The listing builds one solid part. Answer for the finished solid, in the listing's coordinates (mm). Give positions to 0.01 mm unless a question says otherwise; leave off trailing zeros. Write each loop counter-clockwise with the first axis right and the second up, starting at its lowest first coordinate (ties: lowest second). Pieces come first, ordered by that corner, then holes.
```python
from build123d import *

# Parameters (mm, degrees)
SKETCH5_R           = 84.7725
SKETCH5_R_2         = 6.35
BOSS_EXTRUDE1_DEPTH = 6.35


with BuildPart() as part:
    # Sketch5 → Boss-Extrude1 (new body)
    with BuildSketch(Plane(origin=(0, 0, 0), x_dir=(1, 0, 0), z_dir=(0, 1, 0))):
        with BuildLine():
            Line((-108.51132569, 114.857435108), (257.591051155, 114.857435108))
            ThreePointArc((257.591051155, 114.857435108), (263.497362796, 112.410960723), (265.943837181, 106.504649083))
            Line((265.943837181, 106.504649083), (265.943837181, 22.684649083))
            ThreePointArc((265.943837181, 22.684649083), (263.497362796, 16.778337443), (257.591051155, 14.331863057))
            Line((257.591051155, 14.331863057), (240.397032386, 14.331863057))
            ThreePointArc((240.397032386, 14.331863057), (234.490720746, 11.885388672), (232.044246361, 5.979077032))
            Line((232.044246361, 5.979077032), (232.044246361, -98.583895379))
            ThreePointArc((232.044246361, -98.583895379), (229.597771976, -104.490207019), (223.691460335, -106.936681404))
            Line((223.691460335, -106.936681404), (-106.508539665, -106.936681404))
            ThreePointArc((-106.508539665, -106.936681404), (-112.414851305, -104.490207019), (-114.86132569, -98.583895379))
            Line((-114.86132569, -98.583895379), (-114.86132569, 108.507435108))
            ThreePointArc((-114.86132569, 108.507435108), (-113.001453751, 112.997563169), (-108.51132569, 114.857435108))
        make_face()
        Circle(SKETCH5_R, mode=Mode.SUBTRACT)
        with Locations((251.46, 89.968152547)):
            Circle(SKETCH5_R_2, mode=Mode.SUBTRACT)
        with Locations((251.46, 39.221145619)):
            Circle(SKETCH5_R_2, mode=Mode.SUBTRACT)
        with Locations((-95.238376165, -11.844376537)):
            Circle(SKETCH5_R_2, mode=Mode.SUBTRACT)
        with Locations((57.035275027, -75.64676797)):
            Circle(SKETCH5_R_2, mode=Mode.SUBTRACT)
        with Locations((36.152941234, 88.127278006)):
            Circle(SKETCH5_R_2, mode=Mode.SUBTRACT)
    extrude(amount=-BOSS_EXTRUDE1_DEPTH)


solid = part.part
```
Item 1: Consider probe 1 along Z at (x, y) = (251.46, -4.5); probe 2 along Z at (x, y) = (0, -3.5); probe 3 along Z at (x, y) = (35.5, -1.5). Determine where each line is inside the solid, lowest interval first.
Conclusion:
probe 1: z = -114.86 to -96.32, -83.62 to -45.57, -32.87 to -14.33
probe 2: z = -114.86 to -84.77, 84.77 to 106.94
probe 3: z = -114.86 to -94.44, -81.81 to -76.98, 76.98 to 106.94
Item 2: A cutting plane is placed at C-C, the plane z = 0. Give the vertices of the cut face in (x, y), plus the area to 3 significant figures.
Conclusion:
outline: (-114.86, -6.35) - (-84.77, -6.35) - (-84.77, 0) - (-114.86, 0) - close; (84.77, -6.35) - (232.04, -6.35) - (232.04, 0) - (84.77, 0) - close
area: 1,130 mm2
Item 3: A cutting plane is placed at A-A, the plane x = 251.46. Give the vertices of the cut face in (y, z).
Conclusion:
outline: (-6.35, -114.86) - (0, -114.86) - (0, -96.32) - (-6.35, -96.32) - close; (-6.35, -83.62) - (0, -83.62) - (0, -45.57) - (-6.35, -45.57) - close; (-6.35, -32.87) - (0, -32.87) - (0, -14.33) - (-6.35, -14.33) - close
Item 4: A cutting plane is placed at B-B, the plane x = 0. Give the vertices of the cut face in (y, z), plus the area to 3 significant figures.
Conclusion:
outline: (-6.35, -114.86) - (0, -114.86) - (0, -84.77) - (-6.35, -84.77) - close; (-6.35, 84.77) - (0, 84.77) - (0, 106.94) - (-6.35, 106.94) - close
area: 332 mm2
Item 5: Each of these flat-tipped pins is pushed along its axis until it touches: P1, Ø16.5, axis at x = 251.46, z = -39.22, coming from the -Y side; P2, Ø1.9, axis at y = -3, z = 32, coming from the +X side; P3, Ø1.9, axis at x = 245.5, y = -2.5, coming from the +Z side; P4, Ø10, axis at x = 36.15, z = -88.13, coming from the -Y side. Where does it stop, or does it pass through?
Conclusion:
P1: stops at y = -6.35
P2: stops at x = 232.04
P3: stops at z = -14.33
P4: passes through
Item 6: Determine the mould class of faces 1 (the face through (263.43, -3.13, -112.48)), 2 (the face through (234.556, -3.131, -11.95)), 3 (the face through (42.21, -3.13, -90.03)) for opening direction Z: pulls with the +Z half, pulls with the -Z half, needs draft (parallel to the pull), parting line crosses it, or undercut.
Conclusion:
face 1: pulls with the -Z half
face 2: pulls with the +Z half
face 3: undercut
Item 7: A cutting plane is placed at D-D, the plane y = -5.25. Count the separate pieces of the cut face and the enclosed holes in it, plus the area to 3 significant figures.
Conclusion:
separate pieces: 1
enclosed holes: 6
area: 57,100 mm2
